Build history of the part. All positions in model axes, mm. Face numbers are marked on the shaded views. Give positions to 0.01 mm unless a question says otherwise; leave off trailing zeros. Loops run counter-clockwise (first coordinate to the right, second up) from the corner with the lowest first, then second, coordinate; pieces in that order, holes last. Notation, with made-up numbers: M 74.25,-27 L 109.25,-27 A10 cw 109.25,-8 Z; hole C 63,-3.5 d7. An arc over 180 degrees is marked long. Put each result on its own line as item: value.
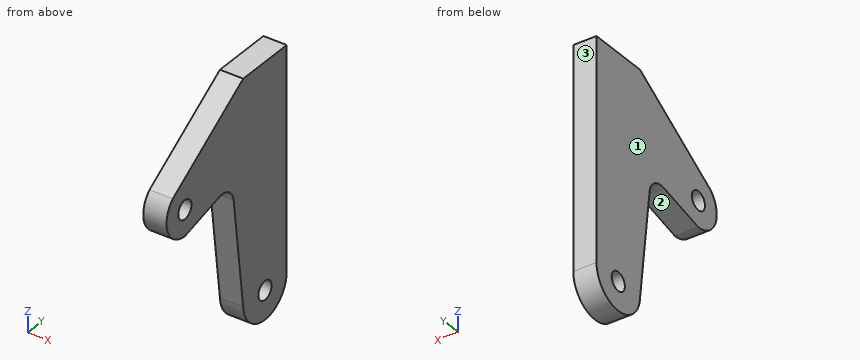
```python
from build123d import *

# Parameters (mm, degrees)
EXTRUDE_1_DEPTH     = 10
SKETCH_2_R          = 4
CUT_EXTRUDE_1_DEPTH = 131.970599025


with BuildPart() as part:
    # Эскиз1 → Вытянуть1 (new body)
    with BuildSketch(Plane(origin=(0, 0, 0), x_dir=(0, 0, -1), z_dir=(1, 0, 0))):
        with BuildLine():
            Line((0, 0), (0, -26.457513111))
            Line((0, -26.457513111), (27.520390874, -69.232651823))
            ThreePointArc((27.520390874, -69.232651823), (39.895894439, -72.361692048), (47.168175164, -61.870842975))
            Line((47.168175164, -61.870842975), (41.925259283, -40.921571184))
            ThreePointArc((41.925259283, -40.921571184), (42.947914526, -35.255861998), (47.872279974, -32.273126802))
            Line((47.872279974, -32.273126802), (95.780101016, -26.457513111))
            ThreePointArc((95.780101016, -26.457513111), (108.222992472, -12.84453329), (94.988313332, 0))
            Line((94.988313332, 0), (0, 0))
        make_face()
    extrude(amount=EXTRUDE_1_DEPTH)

    # Эскиз2 → Вырез-Вытянуть1 (cut, through all)
    with BuildSketch(Plane(origin=(10, 0, 0), x_dir=(0, 0, -1), z_dir=(1, 0, 0))):
        with Locations((95.904397826, -13.228756555)):
            Circle(SKETCH_2_R)
        with Locations((36.015412993, -61.926732738)):
            Circle(SKETCH_2_R)
    extrude(amount=-CUT_EXTRUDE_1_DEPTH, mode=Mode.SUBTRACT)


solid = part.part
```
Q1. Slice it at A-A (y = -16). List the corners of the cut face in (x, z).
Here are the results:
outline: M 0,-107.94 L 10,-107.94 L 10,-98.79 L 0,-98.79 Z; M 0,-93.02 L 10,-93.02 L 10,0 L 0,0 Z
Q2. Mould opens along Y. For the marked faces 1, 2 and 3 say: pulls with the +Y half, pulls with the -Y half, needs draft (parallel to the pull), parting line crosses it, or undercut.
Here are the results:
face 1: needs draft
face 2: undercut
face 3: pulls with the +Y half
Q3. Slice it at C-C (z = -79). List the corners of the cut face in (x, y), and give its area (3 significant figures).
Here are the results:
outline: M 0,-28.49 L 10,-28.49 L 10,0 L 0,0 Z
area: 285 mm²
Q4. Slice it at B-B (x = 6.75). List the corners of the cut face in (y, z).
Here are the results:
outline: M -69.23,-27.52 A11.2 ccw -61.87,-47.17 L -40.92,-41.93 A7 cw -32.27,-47.87 L -26.46,-95.78 A13.24 ccw 0,-94.99 L 0,0 L -26.46,0 Z; hole C -61.93,-36.02 d8; hole C -13.23,-95.9 d8
Q5. Drop flat-ended pins along their axis: pin 1 Ø1.5 at (x, y) = (8, -52) entering from -Z; pin 2 Ø2 at (x, y) = (2.5, -44.5) entering from +Z. Give the stop position or say it passes through.
Here are the results:
pin 1: z = -44.89
pin 2: z = -10.96
Q6. Slice it at D-D (y = -60.5). List the corners of the cut face in (x, z), and give its area (3 significant figures).
Here are the results:
outline: M 0,-46.83 L 10,-46.83 L 10,-39.75 L 0,-39.75 Z; M 0,-32.28 L 10,-32.28 L 10,-21.9 L 0,-21.9 Z
area: 174 mm²
Q7. Probe line 1 (Z direction, x = 8, y = -13); line 2 (Z direction, x = 5.75, y = -11.5); line 3 (Z direction, x = 4.5, y = -40.5). List the from-to ranges inside material, lowest first. Write a range as from..to.
Here are the results:
line 1: -108.23..-99.9, -91.91..0
line 2: -108.11..-99.51, -92.3..0
line 3: -41.83..-9.03
